from build123d import *

# Parameters (mm, degrees)
BOSS_EXTRUDE1_DEPTH      = 19
BOSS_EXTRUDE3_DEPTH      = 60
FILLET1_R                = 10
FILLET2_R                = 10
SKETCH4_R                = 7.5
CUT_EXTRUDE1_DEPTH       = 60
SKETCH6_W                = 60
SKETCH6_H                = 10
BOSS_EXTRUDE4_DEPTH      = 70.5
CUT_EXTRUDE2_DEPTH       = 70.5
BOSS_EXTRUDE6_DEPTH      = 10
BOSS_EXTRUDE6_DEPTH_BACK = 31
SKETCH8_R                = 30
SKETCH10_R               = 10.25
CUT_EXTRUDE3_DEPTH       = 41
SKETCH11_R               = 15
CUT_EXTRUDE4_DEPTH       = 6
CUT_EXTRUDE5_START       = -6
SKETCH12_R               = 15
CUT_EXTRUDE5_DEPTH       = 6
SKETCH13_W               = 10
SKETCH13_H               = 30.419601085
BOSS_EXTRUDE7_DEPTH      = 30
BOSS_EXTRUDE8_DEPTH      = 10


with BuildPart() as part:
    # Sketch1 → Boss-Extrude1 (new body)
    with BuildSketch(Plane(origin=(0, 0, 0), x_dir=(1, 0, 0), z_dir=(0, 1, 0))):
        with BuildLine():
            Line((-20, 0), (-20, -40))
            Line((-20, -40), (20, -40))
            Line((20, -40), (20, 0))
            ThreePointArc((20, 0), (0, 20), (-20, 0))
        make_face()
    extrude(amount=BOSS_EXTRUDE1_DEPTH)

    # Sketch3 → Boss-Extrude3 (add)
    with BuildSketch(Plane(origin=(0, 0, 0), x_dir=(1, 0, 0), z_dir=(0, 1, 0))):
        Polygon((0, -40), (35.25, -40), (35.25, -60), (-35.25, -60), (-35.25, -40), align=None)
    extrude(amount=BOSS_EXTRUDE3_DEPTH)

    # Fillet1
    fillet1_edges = [part.edges().sort_by_distance(p)[0] for p in [
        (20, 9.5, 40),
    ]]
    fillet(fillet1_edges, radius=FILLET1_R)

    # Fillet2
    fillet2_edges = [part.edges().sort_by_distance(p)[0] for p in [
        (-20, 9.5, 40),
    ]]
    fillet(fillet2_edges, radius=FILLET2_R)

    # Sketch4 → Cut-Extrude1 (cut)
    with BuildSketch(Plane.XZ):
        with Locations(Location((0, 0, 0), (0, 0, 270))):
            Circle(SKETCH4_R)
    extrude(amount=-CUT_EXTRUDE1_DEPTH, mode=Mode.SUBTRACT)

    # Sketch6 → Boss-Extrude4 (add)
    with BuildSketch(Plane(origin=(35.25, 0, 0), x_dir=(0, 0, -1), z_dir=(1, 0, 0))):
        with Locations((-90, 55)):
            Rectangle(SKETCH6_W, SKETCH6_H)
    extrude(amount=-BOSS_EXTRUDE4_DEPTH)

    # Sketch7 → Cut-Extrude2 (cut)
    with BuildSketch(Plane(origin=(0, 60, 0), x_dir=(1, 0, 0), z_dir=(0, 1, 0))):
        with BuildLine():
            Line((-30, -120), (30, -120))
            ThreePointArc((30, -120), (0, -90), (-30, -120))
        make_face()
    extrude(amount=-CUT_EXTRUDE2_DEPTH, mode=Mode.SUBTRACT)

    # Sketch8 → Boss-Extrude6 (add, two sides: drawn at the far end of the back side and taken through both)
    with BuildSketch(Plane(origin=(0, 60, 0), x_dir=(1, 0, 0), z_dir=(0, 1, 0)).offset(-BOSS_EXTRUDE6_DEPTH_BACK)):
        with Locations(Location((0, -120, 0), (0, 0, 270))):
            Circle(SKETCH8_R)
    extrude(amount=BOSS_EXTRUDE6_DEPTH + BOSS_EXTRUDE6_DEPTH_BACK)

    # Sketch10 → Cut-Extrude3 (cut)
    with BuildSketch(Plane(origin=(0, 70, 0), x_dir=(1, 0, 0), z_dir=(0, 1, 0))):
        with Locations(Location((0, -120, 0), (0, 0, 270))):
            Circle(SKETCH10_R)
    extrude(amount=-CUT_EXTRUDE3_DEPTH, mode=Mode.SUBTRACT)

    # Sketch11 → Cut-Extrude4 (cut)
    with BuildSketch(Plane(origin=(0, 70, 0), x_dir=(1, 0, 0), z_dir=(0, 1, 0))):
        with Locations(Location((0, -120, 0), (0, 0, 270))):
            Circle(SKETCH11_R)
    extrude(amount=-CUT_EXTRUDE4_DEPTH, mode=Mode.SUBTRACT)

    # Sketch12 → Cut-Extrude5 (cut)
    with BuildSketch(Plane.XZ.offset(-29).offset(CUT_EXTRUDE5_START)):
        with Locations(Location((0, 120, 0), (0, 0, 90))):
            Circle(SKETCH12_R)
    extrude(amount=CUT_EXTRUDE5_DEPTH, mode=Mode.SUBTRACT)

    # Sketch13 → Boss-Extrude7 (add)
    with BuildSketch(Plane.XZ.offset(-29)):
        with Locations((0, 75.209800543)):
            Rectangle(SKETCH13_W, SKETCH13_H)
    extrude(amount=-BOSS_EXTRUDE7_DEPTH)

    # Sketch16 → Boss-Extrude8 (add)
    with BuildSketch(Plane(origin=(5, 0, 0), x_dir=(0, 0, -1), z_dir=(1, 0, 0))):
        Polygon((-90.419601085, 29), (-60, 29), (-60, 0), align=None)
    extrude(amount=-BOSS_EXTRUDE8_DEPTH)


solid = part.part
Read the model definition and answer for the solid it produces. Units are mm, in the model's axes. A direction names the side the tool comes from. Give positions to 0.01 mm unless a question says otherwise; leave off trailing zeros. Write each loop counter-clockwise with the first axis right and the second up, starting at its lowest first coordinate (ties: lowest second). Pieces come first, ordered by that corner, then holes. Notation, with made-up numbers: M 47,4 L 91,4 A9 cw 91,15 Z; hole C 40.5,44.5 d5. An arc over 180 degrees is marked long. One line per item, written item: value. Start each with the question number.
(1) A tool of negligible diameter and unlimited length cuts with its end or side. For faces 1 (the flat face through (20, 25, 60)), 2 (the flat face through (-33, 55, 120)), 3 (the cylindrical face through (-11.49, 49.213, 147.712)), 4 (the flat face through (-3, 64, 130)), 5 (the flat face through (-20, 9, 15)), from which of +Z, -Z, +X, -X, +Y, -Y can it reach the whole face along a straight path? Write none if from no direction.
(2) Find section C-C (z = 82). Determine the outline of the cut face in (x, y).
(3) Find the intervals of material crossed by line 1 (X direction, y = 33, z = 120); line 2 (Y direction, x = 32, z = 118); line 3 (Y direction, x = -3.5, z = 52), in increasing order.
(4) Find section A-A (x = 0). Determine the outline of the cut face in (y, z).
(5) Find section B-B (z = 128). Determine the outline of the cut face in (x, y), plus the area to 3 significant figures.
(6) Flat-ended cylindrical pins translate along their axes: pin 1 Ø5 at (x, z) = (25.5, 38.5) entering from +Y; pin 2 Ø1.6 at (x, y) = (-33, 55.5) entering from +Z; pin 3 Ø18 at (x, z) = (0, 120) entering from -Y; pin 4 Ø5 at (x, y) = (-9.5, 8.5) entering from -Z (3 decimals). Find the tip coordinate at first contact, or state that the pin passes through.
(7) Find section D-D (x = -18). Determine the outline of the cut face in (y, z), plus the area to 3 significant figures.
(8) Determine the mould class of faces 6 (the flat face through (3, 35, 130)), 7 (the flat face through (-20, 25, 60)), 8 (the flat face through (20, 9, 15)) for opening direction X: pulls with the +X half, pulls with the -X half, needs draft (parallel to the pull), parting line crosses it, or undercut.
Results below:
1. face 1: +X, -Y
1. face 2: +Z, -X, +Y, -Y
1. face 3: none
1. face 4: +Y
1. face 5: -Z, -X, +Y, -Y
2. outline: M -35.25,50 L -5,50 L -5,20.97 L 5,20.97 L 5,50 L 35.25,50 L 35.25,60 L -35.25,60 Z
3. line 1: x = -30 to -15, 15 to 30
3. line 2: y = 50 to 60
3. line 3: y = 0 to 60
4. outline: M 0,-20 L 19,-20 L 19,-7.5 L 0,-7.5 Z; M 0,7.5 L 19,7.5 L 19,40 L 60,40 L 60,90 L 70,90 L 70,105 L 64,105 L 64,109.75 L 35,109.75 L 35,105 L 29,105 L 29,90.42 L 0,60 Z; M 29,135 L 35,135 L 35,130.25 L 64,130.25 L 64,135 L 70,135 L 70,150 L 29,150 Z
5. outline: M -28.91,29 L -12.69,29 L -12.69,35 L -6.41,35 L -6.41,64 L -12.69,64 L -12.69,70 L -28.91,70 Z; M 6.41,35 L 12.69,35 L 12.69,29 L 28.91,29 L 28.91,70 L 12.69,70 L 12.69,64 L 6.41,64 Z
5. area: 1,690 mm^2
6. pin 1: stops at y = 60
6. pin 2: stops at z = 120
6. pin 3: passes through
6. pin 4: stops at z = -18.735
7. outline: M 0,-8.72 L 19,-8.72 L 19,40 L 60,40 L 60,96 L 70,96 L 70,144 L 29,144 L 29,96 L 50,96 L 50,60 L 0,60 Z
7. area: 4,450 mm^2
8. face 6: undercut
8. face 7: needs draft
8. face 8: pulls with the +X half
